CAD build for the part. Positions are in the model's coordinates, mm. Face numbers are marked on the shaded views. A direction names the side the tool comes from. Coordinates: 2 decimals unless noted, no trailing zeros. Order: outer loops, then holes, each group sorted by start corner. A loop starts at its lowest first (then second) coordinate and runs counter-clockwise, first axis right, second up. Notation, with made-up numbers: (75, 9) - (100, 9) arc R16 cw to (100, 35) - close; hole circle Ø1 at (29, 57). An arc over 180 degrees is marked (long way). Use one line per item in the form item = value.
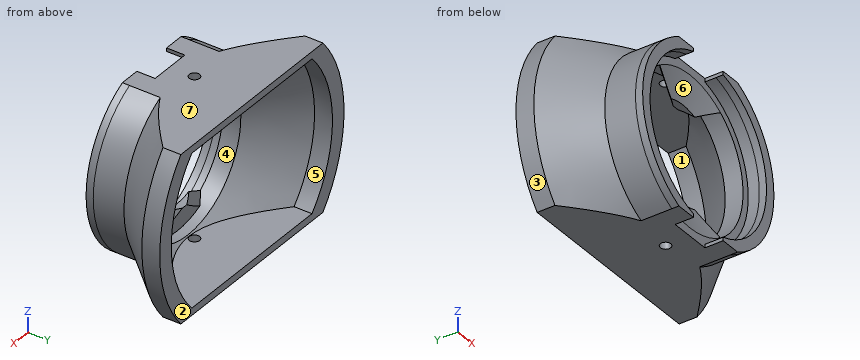
```python
from build123d import *

# Parameters (mm, degrees)
SKETCH2_W           = 56.273883818
SKETCH2_H           = 13.25
CUT_EXTRUDE1_DEPTH  = 58.797058749
BOSS_EXTRUDE2_REACH = 52.486
SKETCH6_W           = 56.273883818
SKETCH6_H           = 2
SKETCH3_W           = 11.78
SKETCH3_H           = 0.962657039
CUT_EXTRUDE2_DEPTH  = 3.1
SKETCH7_R           = 1.45
CUT_EXTRUDE3_DEPTH  = 65.579408483
REVOLVE2_ANGLE      = 70
BOSS_EXTRUDE5_DEPTH = 2
SKETCH16_R          = 13.55
CUT_EXTRUDE6_DEPTH  = 49.961438909
DRAFT11_ANGLE       = -60


with BuildPart() as part:
    # Sketch1 → Revolve1 (revolve)
    with BuildSketch(Plane(origin=(0, 0, 0), x_dir=(0, 0, -1), z_dir=(1, 0, 0)), mode=Mode.PRIVATE) as revolve1_sk:
        Polygon((-26, 0), (-26, 8.590696852), (-36.5, 21), (-36.5, 26), (-31.915197927, 26), (-31.915197927, 21), (-21, 8.1), (-21, 3.1), (-23.0525, 3.1), (-23.0525, 0), align=None)
    revolve(revolve1_sk.sketch.rotate(Axis((0, 0, 0), (0, 1, 0)), 180), axis=Axis((0, 0, 0), (0, 1, 0)))

    # Sketch2 → Cut-Extrude1 (cut, through all)
    with BuildSketch(Plane.XZ):
        with Locations((0, -29.875)):
            Rectangle(SKETCH2_W, SKETCH2_H)
        with Locations((0, 29.875)):
            Rectangle(SKETCH2_W, SKETCH2_H)
    extrude(amount=-CUT_EXTRUDE1_DEPTH, mode=Mode.SUBTRACT)

    # Boss-Extrude2: up to this cone (the profile starts inside it)
    boss_extrude2_end = Plane(origin=(0, 26, 0), z_dir=(0, 1, 0)).offset(-42.718605296) * Cone(1e-06, 111.563900484, 131.850500094, align=(Align.CENTER, Align.CENTER, Align.MIN), mode=Mode.PRIVATE)
    # Sketch6 → Boss-Extrude2 (add, up to the surface)
    with BuildSketch(Plane(origin=(0, 26, 0), x_dir=(1, 0, 0), z_dir=(0, 1, 0)), mode=Mode.PRIVATE) as boss_extrude2_sk1:
        with Locations((0, 22.25)):
            Rectangle(SKETCH6_W, SKETCH6_H)
    boss_extrude2_tool1 = extrude(boss_extrude2_sk1.sketch, amount=-BOSS_EXTRUDE2_REACH, mode=Mode.PRIVATE) & boss_extrude2_end
    add(boss_extrude2_tool1.solids().sort_by_distance((0, 26, -22.25))[0])
    # Sketch6 → Boss-Extrude2 (add, up to the surface)
    with BuildSketch(Plane(origin=(0, 26, 0), x_dir=(1, 0, 0), z_dir=(0, 1, 0)), mode=Mode.PRIVATE) as boss_extrude2_sk2:
        with Locations((0, -22.25)):
            Rectangle(SKETCH6_W, SKETCH6_H)
    boss_extrude2_tool2 = extrude(boss_extrude2_sk2.sketch, amount=-BOSS_EXTRUDE2_REACH, mode=Mode.PRIVATE) & boss_extrude2_end
    add(boss_extrude2_tool2.solids().sort_by_distance((0, 26, 22.25))[0])

    # Sketch3 → Cut-Extrude2 (cut)
    with BuildSketch(Plane.XZ):
        with Locations((0, -22.768671481)):
            Rectangle(SKETCH3_W, SKETCH3_H)
        with Locations((0, 22.768671481)):
            Rectangle(SKETCH3_W, SKETCH3_H)
    extrude(amount=-CUT_EXTRUDE2_DEPTH, mode=Mode.SUBTRACT)

    # Sketch7 → Cut-Extrude3 (cut, through all)
    with BuildSketch(Plane(origin=(0, 0, -23.25), x_dir=(-1, 0, 0), z_dir=(0, 0, -1))):
        with Locations(Location((0, 9.95, 0), (0, 0, 90))):
            Circle(SKETCH7_R)
    extrude(amount=-CUT_EXTRUDE3_DEPTH, mode=Mode.SUBTRACT)

    # Sketch9 → Revolve2 (revolve, symmetric)
    with BuildSketch(Plane(origin=(0, 0, 0), x_dir=(0, 0, -1), z_dir=(1, 0, 0))) as revolve2_sk:
        Polygon((21.518312402, 5.031670845), (21, 3.1), (10.375810352, 5.950718212), (10.894122754, 7.882389057), align=None)
    revolve2 = revolve(axis=Axis((0, 0, 0), (0, 1, 0)), revolution_arc=REVOLVE2_ANGLE / 2)
    revolve2 = revolve2 + revolve(revolve2_sk.sketch, axis=Axis((0, 0, 0), (0, -1, 0)), revolution_arc=REVOLVE2_ANGLE / 2)

    # Mirror3: Revolve2 across plane
    add(revolve2.mirror(Plane.XY))

    # Sketch13 → Boss-Extrude5 (add)
    with BuildSketch(Plane.XZ):
        with BuildLine():
            Line((-5.89, -23.25), (-5.89, -22.287342961))
            ThreePointArc((-5.89, -22.287342961), (-23.0525, 0), (-5.89, 22.287342961))
            Line((-5.89, 22.287342961), (-5.89, 23.25))
            Line((-5.89, 23.25), (-11.637761812, 23.25))
            ThreePointArc((-11.637761812, 23.25), (-26, 0), (-11.637761812, -23.25))
            Line((-11.637761812, -23.25), (-5.89, -23.25))
        make_face()
        with BuildLine():
            Line((5.89, -22.287342961), (5.89, -23.25))
            Line((5.89, -23.25), (11.637761812, -23.25))
            ThreePointArc((11.637761812, -23.25), (26, 0), (11.637761812, 23.25))
            Line((11.637761812, 23.25), (5.89, 23.25))
            Line((5.89, 23.25), (5.89, 22.287342961))
            ThreePointArc((5.89, 22.287342961), (23.0525, 0), (5.89, -22.287342961))
        make_face()
    extrude(amount=BOSS_EXTRUDE5_DEPTH)

    # Sketch16 → Cut-Extrude6 (cut, through all)
    with BuildSketch(Plane.XZ.offset(-3.1)):
        Circle(SKETCH16_R)
    extrude(amount=-CUT_EXTRUDE6_DEPTH, mode=Mode.SUBTRACT)

    # Draft11
    draft11_faces = [part.faces().sort_by_distance(p)[0] for p in [
        (9.908532938, 5.134877582, 14.150851565),
        (-9.908532938, 5.134877582, 14.150851565),
        (9.908532938, 5.134877582, -14.150851565),
        (-9.908532938, 5.134877582, -14.150851565),
    ]]
    draft(draft11_faces, Plane(origin=(0, 3.1, 0), x_dir=(0, 0, -1), z_dir=(0, -1, 0)), DRAFT11_ANGLE)


solid = part.part
```
Item 1: Drill centre lines: line 1 (Z direction, x = 5.5, y = 18.25); line 2 (X direction, y = 8.5, z = -17.5). Where is each one in solid material? Low to high. Write a range as [from, to].
Derived:
line_1 = [-23.25, -21.25], [21.25, 23.25]
line_2 = [-19.23, -12.21], [12.21, 19.23]
Item 2: Drop flat-ended pins along their axis: pin 1 (8 mm diameter, centred on x = 18, z = 12.5, fed in from +Y); pin 2 (8 mm diameter, centred on x = 9, z = 16, fed in from +Y); pin 3 (5 mm diameter, centred on y = 2, z = 3.5, fed in from -X); pin 4 (2.5 mm diameter, centred on x = 0, y = 9.95, fed in from +Z). Give the stop position or say it passes through.
Derived:
pin_1 = 13.91
pin_2 = 9.7
pin_3 = -25.98
pin_4 = through
Item 3: Cut at A-A, the plane x = 0. Write the cut outline in (y, z), plus the area to 3 significant figures.
Derived:
outline = (3.1, -23.25) - (8.5, -23.25) - (8.5, -21.25) - (8.4, -21.25) - (8.1, -21) - (5.17, -21) - (7.17, -13.55) - (5.1, -13.55) - (3.1, -21) - close; (3.1, 21) - (5.1, 13.55) - (7.17, 13.55) - (5.17, 21) - (8.1, 21) - (8.4, 21.25) - (8.5, 21.25) - (8.5, 23.25) - (3.1, 23.25) - close; (11.4, -23.25) - (26, -23.25) - (26, -21.25) - (11.4, -21.25) - close; (11.4, 21.25) - (26, 21.25) - (26, 23.25) - (11.4, 23.25) - close
area = 113 mm²
Item 4: Two-plate mould, pull along X, no slides. Class the marked faces 1, 2, 3 and 4: +X half, -X half, draft (parallel to the pull), parting line (faces both ways), or undercut.
Derived:
face_1 = undercut
face_2 = draft
face_3 = -X half
face_4 = undercut
Item 5: Cut at B-B, the plane z = 0. Write the cut outline in (x, y), plus the area to 3 significant figures.
Derived:
outline = (-36.5, 21) - (-26, 8.59) - (-26, -2) - (-23.05, -2) - (-23.05, 3.1) - (-21, 3.1) - (-21, 8.1) - (-31.92, 21) - (-31.92, 26) - (-36.5, 26) - close; (21, 3.1) - (23.05, 3.1) - (23.05, -2) - (26, -2) - (26, 8.59) - (36.5, 21) - (36.5, 26) - (31.92, 26) - (31.92, 21) - (21, 8.1) - close
area = 244 mm²
Item 6: Cut at C-C, the plane y = 9.95. Write the cut outline in (x, z).
Derived:
outline = (-14.02, -23.25) - (-1.45, -23.25) - (-1.45, -21.25) - (-7.59, -21.25) arc R22.57 cw to (-7.59, 21.25) - (-1.45, 21.25) - (-1.45, 23.25) - (-14.02, 23.25) arc R27.15 ccw to start; (1.45, -23.25) - (14.02, -23.25) arc R27.15 ccw to (14.02, 23.25) - (1.45, 23.25) - (1.45, 21.25) - (7.59, 21.25) arc R22.57 cw to (7.59, -21.25) - (1.45, -21.25) - close
Item 7: 3-axis set-ups, long thin cutter, end or side, ignore diameter. For the marked faces 5, 6 and 7: which of +Z, -Z, +X, -X, +Y, -Y reach the whole face in a straight line?
Derived:
face_5 = +Y
face_6 = -Y
face_7 = +Z, +X, -X, +Y, -Y
